Geometry check sheet. Reference: the model listing, model coordinates, mm. Coordinates: 2 decimals unless noted, no trailing zeros. Write each loop counter-clockwise with the first axis right and the second up, starting at its lowest first coordinate (ties: lowest second). Pieces come first, ordered by that corner, then holes. Notation, with made-up numbers: (73, -5) -> (120, -5) arc R25 cw to (120, 24) -> close; hole circle Ø6 at (57.25, 10.25). An arc over 180 degrees is marked (long way). Answer in a Markdown table with one row per item. Add a question column.
1. Cross-section at B-B on x = 120.5. Record the cut outline in (y, z), and give its area (3 significant figures).
2. Cross-section at C-C on z = 3.25. Give the number of separate pieces and of enclosed holes in the cut face, and give its area (3 significant figures).
3. Scan lines: L1, parallel to Y at x = 175, z = 6.25; L2, parallel to X at y = 35, z = 5; L3, parallel to X at y = 3, z = 9.75. Record each from-to range of solid material in increasing order. Write a range as from..to.
4. Cross-section at A-A on y = 47. Record the cut outline in (x, z).
5. Depth check by flat-ended pin: P1, Ø21, axis at x = -175, y = 0, coming from the +Z side. Enter the tip coordinate at first touch or a pass-through.
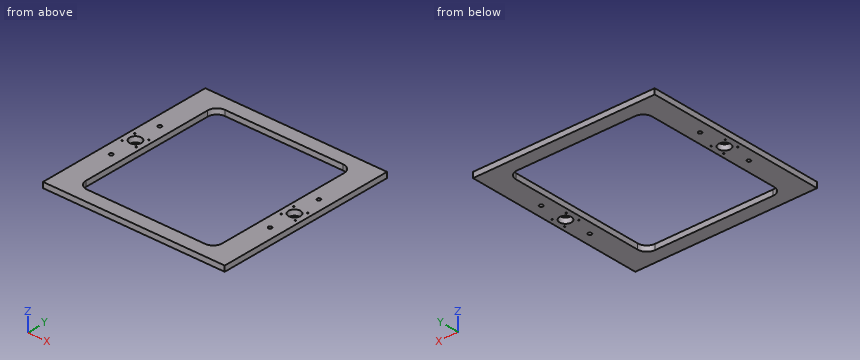
```python
from build123d import *

# Parameters (mm, degrees)
F0_W     = 400
F0_H     = 400
F0_R     = 4
F0_R_2   = 1.5
F0_R_3   = 13
F1_DEPTH = 12


with BuildPart() as f1:
    # F0 (on Top) → F1 (new body)
    with BuildSketch(Plane.XY):
        Rectangle(F0_W, F0_H)
        with Locations((-175, -60)):
            Circle(F0_R, mode=Mode.SUBTRACT)
        with Locations((-190.5, -15.5)):
            Circle(F0_R_2, mode=Mode.SUBTRACT)
        with Locations((-159.5, -15.5)):
            Circle(F0_R_2, mode=Mode.SUBTRACT)
        with Locations((175, -60)):
            Circle(F0_R, mode=Mode.SUBTRACT)
        with Locations((159.626022, -15.5)):
            Circle(F0_R_2, mode=Mode.SUBTRACT)
        with Locations((190.626022, -15.5)):
            Circle(F0_R_2, mode=Mode.SUBTRACT)
        with Locations((-190.5, 15.5)):
            Circle(F0_R_2, mode=Mode.SUBTRACT)
        with Locations((-175, 0)):
            Circle(F0_R_3, mode=Mode.SUBTRACT)
        with Locations((-159.5, 15.5)):
            Circle(F0_R_2, mode=Mode.SUBTRACT)
        with Locations((-175, 60)):
            Circle(F0_R, mode=Mode.SUBTRACT)
        with BuildLine():
            Line((-130, 170), (130, 170))
            ThreePointArc((130, 170), (144.142136, 164.142136), (150, 150))
            Line((150, 150), (150, -150))
            ThreePointArc((150, -150), (144.142136, -164.142136), (130, -170))
            Line((130, -170), (-130, -170))
            ThreePointArc((-130, -170), (-144.142136, -164.142136), (-150, -150))
            Line((-150, -150), (-150, 150))
            ThreePointArc((-150, 150), (-144.142136, 164.142136), (-130, 170))
        make_face(mode=Mode.SUBTRACT)
        with Locations((159.5, 15.5)):
            Circle(F0_R_2, mode=Mode.SUBTRACT)
        with Locations((175, 0)):
            Circle(F0_R_3, mode=Mode.SUBTRACT)
        with Locations((190.5, 15.5)):
            Circle(F0_R_2, mode=Mode.SUBTRACT)
        with Locations((175, 60)):
            Circle(F0_R, mode=Mode.SUBTRACT)
    extrude(amount=F1_DEPTH)


solid = f1.part
```
Results found:
| question | item | result |
|---|---|---|
| 1 | outline | (-200, 0) -> (-170, 0) -> (-170, 12) -> (-200, 12) -> close; (170, 0) -> (200, 0) -> (200, 12) -> (170, 12) -> close |
| 1 | area | 720 mm^2 |
| 2 | separate pieces | 1 |
| 2 | enclosed holes | 15 |
| 2 | area | 57,000 mm^2 |
| 3 | L1 | y = -200..-64, -56..-13, 13..56, 64..200 |
| 3 | L2 | x = -200..-150, 150..200 |
| 3 | L3 | x = -200..-187.65, -162.35..-150, 150..162.35, 187.65..200 |
| 4 | outline | (-200, 0) -> (-150, 0) -> (-150, 12) -> (-200, 12) -> close; (150, 0) -> (200, 0) -> (200, 12) -> (150, 12) -> close |
| 5 | P1 | passes through |
